```python
from build123d import *

# Parameters (mm, degrees)
SKETCH2_R               = 98.425
BOSS_EXTRUDE1_DEPTH     = 12.7
SKETCH3_R               = 9.525
CUT_EXTRUDE4_DEPTH      = 12.7
CUT_EXTRUDE4_DEPTH_BACK = 12.7
CUT_EXTRUDE9_START      = -2.54
SKETCH5_R               = 3.175
CUT_EXTRUDE9_DEPTH      = 15.24
CIRPATTERN1_COUNT       = 12
SKETCH6_R               = 9.525
BOSS_EXTRUDE2_DEPTH     = 12.7
CUT_EXTRUDE10_START     = -12.7
SKETCH8_R               = 3.175
CUT_EXTRUDE10_DEPTH     = 15.24
CIRPATTERN2_COUNT       = 4


with BuildPart() as part:
    # Sketch2 → Boss-Extrude1 (new body)
    with BuildSketch(Plane(origin=(0, 0, 0), x_dir=(1, 0, 0), z_dir=(0, 1, 0))):
        Circle(SKETCH2_R)
    extrude(amount=BOSS_EXTRUDE1_DEPTH)

    # Sketch3 → Cut-Extrude4 (cut, two sides)
    with BuildSketch(Plane(origin=(0, 0, 0), x_dir=(1, 0, 0), z_dir=(0, 1, 0))) as cut_extrude4_sk:
        Circle(SKETCH3_R)
    extrude(amount=CUT_EXTRUDE4_DEPTH, mode=Mode.SUBTRACT)
    extrude(cut_extrude4_sk.sketch, amount=-CUT_EXTRUDE4_DEPTH_BACK, mode=Mode.SUBTRACT)

    # Sketch5 → Cut-Extrude9 (cut)
    with BuildSketch(Plane(origin=(0, 0, 0), x_dir=(1, 0, 0), z_dir=(0, 1, 0)).offset(CUT_EXTRUDE9_START)):
        with Locations((0, -92.202)):
            Circle(SKETCH5_R)
    cut_extrude9 = extrude(amount=CUT_EXTRUDE9_DEPTH, mode=Mode.SUBTRACT)

    # CirPattern1: Cut-Extrude9 ×12 about axis
    cirpattern1_axis = Axis((0, 0, 0), (0, 1, 0))
    for i in range(1, CIRPATTERN1_COUNT):
        add(cut_extrude9.rotate(cirpattern1_axis, i * 360 / CIRPATTERN1_COUNT), mode=Mode.SUBTRACT)

    # Sketch6 → Boss-Extrude2 (add)
    with BuildSketch(Plane(origin=(0, 0, 0), x_dir=(-1, 0, 0), z_dir=(0, 1, 0))):
        with Locations((62.861792847, 62.861792847)):
            Circle(SKETCH6_R)
    boss_extrude2 = extrude(amount=-BOSS_EXTRUDE2_DEPTH)

    # Sketch8 → Cut-Extrude10 (cut)
    with BuildSketch(Plane(origin=(0, 0, 0), x_dir=(1, 0, 0), z_dir=(0, 1, 0)).offset(CUT_EXTRUDE10_START)):
        with Locations((-62.861792847, -62.861792847)):
            Circle(SKETCH8_R)
    cut_extrude10 = extrude(amount=CUT_EXTRUDE10_DEPTH, mode=Mode.SUBTRACT)

    # CirPattern2: Boss-Extrude2, Cut-Extrude10 ×4 about axis
    cirpattern2_axis = Axis((0, 0, 0), (0, 1, 0))
    for i in range(1, CIRPATTERN2_COUNT):
        add(boss_extrude2.rotate(cirpattern2_axis, i * 360 / CIRPATTERN2_COUNT))
        add(cut_extrude10.rotate(cirpattern2_axis, i * 360 / CIRPATTERN2_COUNT), mode=Mode.SUBTRACT)


solid = part.part
```
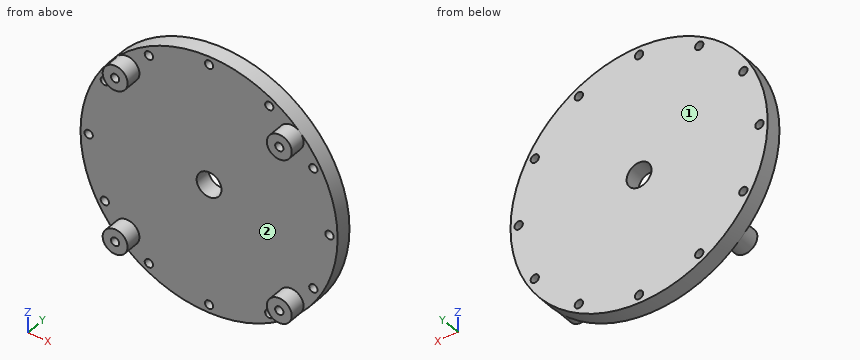
For this review, take the finished solid that the model builds, in its own axes (mm). Face numbers are marked on the shaded views. Round coordinates to 2 decimals unless told otherwise and drop trailing zeros. Loops run counter-clockwise (first coordinate to the right, second up) from the corner with the lowest first, then second, coordinate; pieces in that order, holes last.
(1) We need section C-C (y = -7). Give the boundary of the cut face in (x, z) (3 decimals).
Returned:
outline: circle Ø19.05 at (-62.862, -62.862); circle Ø19.05 at (-62.862, 62.862); circle Ø19.05 at (62.862, -62.862); circle Ø19.05 at (62.862, 62.862); hole circle Ø6.35 at (-62.862, -62.862); hole circle Ø6.35 at (-62.862, 62.862); hole circle Ø6.35 at (62.862, -62.862); hole circle Ø6.35 at (62.862, 62.862)
(2) We need section B-B (x = 0). Give the boundary of the cut face in (y, z) (3 decimals).
Returned:
outline: (0, -98.425) - (12.7, -98.425) - (12.7, -95.377) - (0, -95.377) - close; (0, -89.027) - (12.7, -89.027) - (12.7, -9.525) - (0, -9.525) - close; (0, 9.525) - (12.7, 9.525) - (12.7, 89.027) - (0, 89.027) - close; (0, 95.377) - (12.7, 95.377) - (12.7, 98.425) - (0, 98.425) - close
(3) Clearance check with flat-ended pins moving along their axes: P1, Ø5.5, axis at x = 0, z = 92.202, coming from the +Y side; P2, Ø4, axis at x = 42.5, z = -41.5, coming from the -Y side; P3, Ø1.5, axis at x = -48, y = 9.5, coming from the +Z side; P4, Ø8, axis at x = -53.5, y = -7, coming from the -Z side. State where each tip first meets the part, or that it passes through.
Returned:
P1: passes through
P2: stops at y = 0
P3: stops at z = 86.34
P4: stops at z = -70.73
(4) We need section A-A (z = 0). Give the boundary of the cut face in (x, y) (3 decimals), plus the area to 3 significant figures.
Returned:
outline: (-98.425, 0) - (-95.377, 0) - (-95.377, 12.7) - (-98.425, 12.7) - close; (-89.027, 0) - (-9.525, 0) - (-9.525, 12.7) - (-89.027, 12.7) - close; (9.525, 0) - (89.027, 0) - (89.027, 12.7) - (9.525, 12.7) - close; (95.377, 0) - (98.425, 0) - (98.425, 12.7) - (95.377, 12.7) - close
area: 2,100 mm2
(5) Mouldability with a two-part tool opening along X and no side actions: class the marked faces 1 and 2 as released by +X, released by -X, zero draft, split by the parting line, or undercut.
Returned:
face 1: zero draft
face 2: undercut
(6) Wall thickness on line 1 along X through (y, z) = (5.5, 0) (3 decimals); line 2 along Z through (x, y) = (-78.5, 3.5): over which ranges is each line inside the solid? List them lowest first.
Returned:
line 1: x = -98.425 to -95.377, -89.027 to -9.525, 9.525 to 89.027, 95.377 to 98.425
line 2: z = -59.37 to -48.98, -43.23 to 43.23, 48.98 to 59.37
(7) We need section D-D (z = -57). Give the boundary of the cut face in (x, y).
Returned:
outline: (-80.24, 0) - (-70.37, 0) - (-70.37, -12.7) - (-55.35, -12.7) - (-55.35, 0) - (55.35, 0) - (55.35, -12.7) - (70.37, -12.7) - (70.37, 0) - (80.24, 0) - (80.24, 12.7) - (-80.24, 12.7) - close
